from build123d import *

# Parameters (mm, degrees)
F0_R      = 20
F0_R_2    = 5
F1_DEPTH  = 55
F2_R      = 9.25
F3_DEPTH  = 12
F4_R      = 6.25
F5_DEPTH  = 13
F6_SIZE   = 1
F7_R      = 1.5
F8_DEPTH  = 20.001
F9_SIZE   = 2
F10_R     = 1.5
F11_DEPTH = 10


with BuildPart() as f1:
    # F0 (on Top) → F1 (new body)
    with BuildSketch(Plane.XY):
        Circle(F0_R)
        Circle(F0_R_2, mode=Mode.SUBTRACT)
    extrude(amount=F1_DEPTH)

    # F2 (on face) → F3 (cut)
    with BuildSketch(Plane.XY.offset(55)):
        Circle(F2_R)
    extrude(amount=-F3_DEPTH, mode=Mode.SUBTRACT)

    # F4 (on face) → F5 (cut)
    with BuildSketch(Plane.XY.offset(43)):
        Circle(F4_R)
    extrude(amount=-F5_DEPTH, mode=Mode.SUBTRACT)

    # F6
    f6_edges = [f1.edges().sort_by_distance(p)[0] for p in [
        (-9.25, 0, 55),
        (-20, 0, 55),
    ]]
    chamfer(f6_edges, length=F6_SIZE)

    # F7 (on Front) → F8 (cut, through all)
    with BuildSketch(Plane.XZ):
        with Locations((0, 52)):
            Circle(F7_R)
    extrude(amount=F8_DEPTH, mode=Mode.SUBTRACT)

    # F9
    f9_edges = [f1.edges().sort_by_distance(p)[0] for p in [
        (-5, 0, 0),
    ]]
    chamfer(f9_edges, length=F9_SIZE)

    # F10 (on face) → F11 (cut)
    with BuildSketch(Plane(origin=(0, 0, 0), x_dir=(1, 0, 0), z_dir=(0, 0, -1))):
        with Locations((-16, 0)):
            Circle(F10_R)
        with Locations((0, 16)):
            Circle(F10_R)
        with Locations((16, 0)):
            Circle(F10_R)
        with Locations((0, -16)):
            Circle(F10_R)
    extrude(amount=-F11_DEPTH, mode=Mode.SUBTRACT)


solid = f1.part
Build history of the part. All positions in model axes, mm. A direction names the side the tool comes from. Give positions to 0.01 mm unless a question says otherwise; leave off trailing zeros. Order: outer loops, then holes, each group sorted by start corner. A loop starts at its lowest first (then second) coordinate and runs counter-clockwise, first axis right, second up. Notation, with made-up numbers: M 28.25,-14.5 L 71.25,-14.5 A19 ccw 71.25,13.5 Z; hole C 10.5,89.5 d10. An arc over 180 degrees is marked long. Use one line per item in the form item = value.
Q1. Wall check: probe 1 along Y at (x, z) = (0, 48); probe 2 along Y at (x, z) = (0, 33); probe 3 along Z at (x, y) = (-2.5, 7). Give the ranges that are in metal, low to high.
Conclusion:
probe_1 = -20 to -9.25, 9.25 to 20
probe_2 = -20 to -6.25, 6.25 to 20
probe_3 = 0 to 43
Q2. Slice it at B-B, the plane z = 49.5. Write the cut outline in (x, y).
Conclusion:
outline = C 0,0 d40; hole C 0,0 d18.5
Q3. Slice it at A-A, the plane x = 0. State how many separate pieces and enclosed holes the cut face has, and give its area (3 significant figures).
Conclusion:
separate_pieces = 3
enclosed_holes = 0
area = 1,420 mm2
Q4. Pull direction Y, two halves, no side cores. Call faces 3 (the cylindrical face through (-1.11, -17.01, 4.93)), 4 (the cylindrical face through (-4.336, -19.524, 26.622)), 5 (the flat face through (0, -9, 0)), 6 (the cylindrical face through (-1.08, -4.88, 15.8)): released by +Y, released by -Y, zero draft, split by the parting line, or undercut.
Conclusion:
face_3 = undercut
face_4 = split by the parting line
face_5 = zero draft
face_6 = undercut
Q5. Slice it at C-C, the plane z = 22.5. Write the cut outline in (x, y).
Conclusion:
outline = C 0,0 d40; hole C 0,0 d10
Q6. Pin check, flat tips, straight feed: P1, Ø11, axis at x = 0, y = 0, coming from the +Z side; P2, Ø8, axis at x = 8, z = 39, coming from the +Y side; P3, Ø5, axis at x = 0, z = 52, coming from the +Y side. Stop position of each tip, or through.
Conclusion:
P1 = 30
P2 = 19.6
P3 = 20
Q7. Which spindle directions (+Z, -Z, +X, -X, +Y, -Y) get a long thin tool onto all of the face, cutting with end or side? Do faces 1 (the cylindrical face through (14.5, -0.07, 4.93)), 2 (the flat face through (6.04, 2.19, 43)). Say none if no direction does.
Conclusion:
face_1 = -Z
face_2 = +Z
